Autodesk Inventor part; units mm, degrees
ref_plane "IP_2_XY" through (15.5, 0, 0) normal (1, 0, 0) x (0, 0, -1)
ref_plane "IP_2_YZ" through (15.5, 0, 0) normal (0, 0, -1) x (0, 1, 0)
ref_plane "IP_2_ZX" through (15.5, 0, 0) normal (0, 1, 0) x (1, 0, 0)
sketch "Sketch_1" plane through (0, 0, 0) normal (0, 0, 1) x (1, 0, 0)
  line L0 (50, 0) -> (-50, 0)
  line L1 (0, 23.1136) -> (0, 17.5)
  line L2 (0, 17.5) -> (31, 17.5)
  line L3 (31, 17.5) -> (31, 23.1136)
  line L4 (31, 23.1136) -> (27.7302, 23.1136)
  arc A0 (27.7302, 23.1136) -> (26.8226, 22.8599) centre (27.7302, 21.3636) ccw
  arc A1 (19.6774, 22.8599) -> (26.8226, 22.8599) centre (23.25, 28.75) ccw
  arc A2 (19.6774, 22.8599) -> (18.7698, 23.1136) centre (18.7698, 21.3636) ccw
  line L5 (18.7698, 23.1136) -> (12.2302, 23.1136)
  arc A3 (12.2302, 23.1136) -> (11.3226, 22.8599) centre (12.2302, 21.3636) ccw
  arc A4 (4.1774, 22.8599) -> (11.3226, 22.8599) centre (7.75, 28.75) ccw
  arc A5 (4.1774, 22.8599) -> (3.2698, 23.1136) centre (3.2698, 21.3636) ccw
  line L6 (3.2698, 23.1136) -> (0, 23.1136)
revolve "Revolution1" add sketch "Sketch_1" angle 360 about axis through (50, 0, 0) along (1, 0, 0)
ref_plane "IP_2_XY" through (15.5, 0, 0) normal (1, 0, 0) x (0, 0, -1)
ref_plane "IP_2_YZ" through (15.5, 0, 0) normal (0, 0, -1) x (0, 1, 0)
ref_plane "IP_2_ZX" through (15.5, 0, 0) normal (0, 1, 0) x (1, 0, 0)
ref_plane "IP_3_1_XY" through (7.75, 28.75, 0) normal (1, 0, 0) x (0, 0, -1)
ref_plane "IP_3_1_YZ" through (7.75, 28.75, 0) normal (0, 0, -1) x (0, 1, 0)
ref_plane "IP_3_1_ZX" through (7.75, 28.75, 0) normal (0, 1, 0) x (1, 0, 0)
ref_plane "IP_3_10_XY" through (7.75, 23.2592, -16.8988) normal (1, 0, 0) x (0, 0, -1)
ref_plane "IP_3_10_YZ" through (7.75, 23.2592, -16.8988) normal (0, 0, -1) x (0, 1, 0)
ref_plane "IP_3_10_ZX" through (7.75, 23.2592, -16.8988) normal (0, 1, 0) x (1, 0, 0)
ref_plane "IP_3_2_XY" through (7.75, 23.2592, 16.8988) normal (1, 0, 0) x (0, 0, -1)
ref_plane "IP_3_2_YZ" through (7.75, 23.2592, 16.8988) normal (0, 0, -1) x (0, 1, 0)
ref_plane "IP_3_2_ZX" through (7.75, 23.2592, 16.8988) normal (0, 1, 0) x (1, 0, 0)
ref_plane "IP_3_3_XY" through (7.75, 8.8842, 27.3429) normal (1, 0, 0) x (0, 0, -1)
ref_plane "IP_3_3_YZ" through (7.75, 8.8842, 27.3429) normal (0, 0, -1) x (0, 1, 0)
ref_plane "IP_3_3_ZX" through (7.75, 8.8842, 27.3429) normal (0, 1, 0) x (1, 0, 0)
ref_plane "IP_3_4_XY" through (7.75, -8.8842, 27.3429) normal (1, 0, 0) x (0, 0, -1)
ref_plane "IP_3_4_YZ" through (7.75, -8.8842, 27.3429) normal (0, 0, -1) x (0, 1, 0)
ref_plane "IP_3_4_ZX" through (7.75, -8.8842, 27.3429) normal (0, 1, 0) x (1, 0, 0)
ref_plane "IP_3_5_XY" through (7.75, -23.2592, 16.8988) normal (1, 0, 0) x (0, 0, -1)
ref_plane "IP_3_5_YZ" through (7.75, -23.2592, 16.8988) normal (0, 0, -1) x (0, 1, 0)
ref_plane "IP_3_5_ZX" through (7.75, -23.2592, 16.8988) normal (0, 1, 0) x (1, 0, 0)
ref_plane "IP_3_6_XY" through (7.75, -28.75, 0) normal (1, 0, 0) x (0, 0, -1)
ref_plane "IP_3_6_YZ" through (7.75, -28.75, 0) normal (0, 0, -1) x (0, 1, 0)
ref_plane "IP_3_6_ZX" through (7.75, -28.75, 0) normal (0, 1, 0) x (1, 0, 0)
ref_plane "IP_3_7_XY" through (7.75, -23.2592, -16.8988) normal (1, 0, 0) x (0, 0, -1)
ref_plane "IP_3_7_YZ" through (7.75, -23.2592, -16.8988) normal (0, 0, -1) x (0, 1, 0)
ref_plane "IP_3_7_ZX" through (7.75, -23.2592, -16.8988) normal (0, 1, 0) x (1, 0, 0)
ref_plane "IP_3_8_XY" through (7.75, -8.8842, -27.3429) normal (1, 0, 0) x (0, 0, -1)
ref_plane "IP_3_8_YZ" through (7.75, -8.8842, -27.3429) normal (0, 0, -1) x (0, 1, 0)
ref_plane "IP_3_8_ZX" through (7.75, -8.8842, -27.3429) normal (0, 1, 0) x (1, 0, 0)
ref_plane "IP_3_9_XY" through (7.75, 8.8842, -27.3429) normal (1, 0, 0) x (0, 0, -1)
ref_plane "IP_3_9_YZ" through (7.75, 8.8842, -27.3429) normal (0, 0, -1) x (0, 1, 0)
ref_plane "IP_3_9_ZX" through (7.75, 8.8842, -27.3429) normal (0, 1, 0) x (1, 0, 0)
ref_plane "IP_4_1_XY" through (23.25, 27.3429, 8.8842) normal (1, 0, 0) x (0, 0, -1)
ref_plane "IP_4_1_YZ" through (23.25, 27.3429, 8.8842) normal (0, 0, -1) x (0, 1, 0)
ref_plane "IP_4_1_ZX" through (23.25, 27.3429, 8.8842) normal (0, 1, 0) x (1, 0, 0)
ref_plane "IP_4_10_XY" through (23.25, 27.3429, -8.8842) normal (1, 0, 0) x (0, 0, -1)
ref_plane "IP_4_10_YZ" through (23.25, 27.3429, -8.8842) normal (0, 0, -1) x (0, 1, 0)
ref_plane "IP_4_10_ZX" through (23.25, 27.3429, -8.8842) normal (0, 1, 0) x (1, 0, 0)
ref_plane "IP_4_2_XY" through (23.25, 16.8988, 23.2592) normal (1, 0, 0) x (0, 0, -1)
ref_plane "IP_4_2_YZ" through (23.25, 16.8988, 23.2592) normal (0, 0, -1) x (0, 1, 0)
ref_plane "IP_4_2_ZX" through (23.25, 16.8988, 23.2592) normal (0, 1, 0) x (1, 0, 0)
ref_plane "IP_4_3_XY" through (23.25, 0, 28.75) normal (1, 0, 0) x (0, 0, -1)
ref_plane "IP_4_3_YZ" through (23.25, 0, 28.75) normal (0, 0, -1) x (0, 1, 0)
ref_plane "IP_4_3_ZX" through (23.25, 0, 28.75) normal (0, 1, 0) x (1, 0, 0)
ref_plane "IP_4_4_XY" through (23.25, -16.8988, 23.2592) normal (1, 0, 0) x (0, 0, -1)
ref_plane "IP_4_4_YZ" through (23.25, -16.8988, 23.2592) normal (0, 0, -1) x (0, 1, 0)
ref_plane "IP_4_4_ZX" through (23.25, -16.8988, 23.2592) normal (0, 1, 0) x (1, 0, 0)
ref_plane "IP_4_5_XY" through (23.25, -27.3429, 8.8842) normal (1, 0, 0) x (0, 0, -1)
ref_plane "IP_4_5_YZ" through (23.25, -27.3429, 8.8842) normal (0, 0, -1) x (0, 1, 0)
ref_plane "IP_4_5_ZX" through (23.25, -27.3429, 8.8842) normal (0, 1, 0) x (1, 0, 0)
ref_plane "IP_4_6_XY" through (23.25, -27.3429, -8.8842) normal (1, 0, 0) x (0, 0, -1)
ref_plane "IP_4_6_YZ" through (23.25, -27.3429, -8.8842) normal (0, 0, -1) x (0, 1, 0)
ref_plane "IP_4_6_ZX" through (23.25, -27.3429, -8.8842) normal (0, 1, 0) x (1, 0, 0)
ref_plane "IP_4_7_XY" through (23.25, -16.8988, -23.2592) normal (1, 0, 0) x (0, 0, -1)
ref_plane "IP_4_7_YZ" through (23.25, -16.8988, -23.2592) normal (0, 0, -1) x (0, 1, 0)
ref_plane "IP_4_7_ZX" through (23.25, -16.8988, -23.2592) normal (0, 1, 0) x (1, 0, 0)
ref_plane "IP_4_8_XY" through (23.25, 0, -28.75) normal (1, 0, 0) x (0, 0, -1)
ref_plane "IP_4_8_YZ" through (23.25, 0, -28.75) normal (0, 0, -1) x (0, 1, 0)
ref_plane "IP_4_8_ZX" through (23.25, 0, -28.75) normal (0, 1, 0) x (1, 0, 0)
ref_plane "IP_4_9_XY" through (23.25, 16.8988, -23.2592) normal (1, 0, 0) x (0, 0, -1)
ref_plane "IP_4_9_YZ" through (23.25, 16.8988, -23.2592) normal (0, 0, -1) x (0, 1, 0)
ref_plane "IP_4_9_ZX" through (23.25, 16.8988, -23.2592) normal (0, 1, 0) x (1, 0, 0)
properties part number "hpc_Q2307-ACC_2"
Work out the finished part from the listing and answer in its coordinate system (mm). Give positions to 0.01 mm unless a question says otherwise; leave off trailing zeros. Write each loop counter-clockwise with the first axis right and the second up, starting at its lowest first coordinate (ties: lowest second). Pieces come first, ordered by that corner, then holes.
(1) The part is cut by section C-C on x = 16. Write down the section's boundary in (y, z).
Final values:
outline: circle Ø46.23 at (0, 0); hole circle Ø35 at (0, 0)
(2) The mould has two halves that part along Y. Classify faces 1 (the flat face through (31, 8, 16)), 2 (the cylindrical face through (29.342, -5.011, 22.564)), 3 (the cylindrical face through (15.717, -13.887, -10.648)): pulls with the +Y half, pulls with the -Y half, needs draft (parallel to the pull), parting line crosses it, or undercut.
Final values:
face 1: needs draft
face 2: parting line crosses it
face 3: undercut
(3) The part is cut by section A-A on y = 0. Write down the section's boundary in (x, z).
Final values:
outline: (0, -23.11) - (3.27, -23.11) arc R1.75 ccw to (4.18, -22.86) arc R6.89 cw to (11.32, -22.86) arc R1.75 ccw to (12.23, -23.11) - (18.77, -23.11) arc R1.75 ccw to (19.68, -22.86) arc R6.89 cw to (26.82, -22.86) arc R1.75 ccw to (27.73, -23.11) - (31, -23.11) - (31, -17.5) - (0, -17.5) - close; (0, 17.5) - (31, 17.5) - (31, 23.11) - (27.73, 23.11) arc R1.75 ccw to (26.82, 22.86) arc R6.89 cw to (19.68, 22.86) arc R1.75 ccw to (18.77, 23.11) - (12.23, 23.11) arc R1.75 ccw to (11.32, 22.86) arc R6.89 cw to (4.18, 22.86) arc R1.75 ccw to (3.27, 23.11) - (0, 23.11) - close
(4) The part is cut by section D-D on x = 6.5. Write down the section's boundary in (y, z), plus the area to 3 significant figures.
Final values:
outline: circle Ø43.95 at (0, 0); hole circle Ø35 at (0, 0)
area: 555 mm2
(5) Flat-ended cylindrical pins translate along their axes: pin 1 Ø5 at (x, y) = (21.5, 15.5) entering from +Z; pin 2 Ø4 at (x, y) = (9.5, -9) entering from -Z; pin 3 Ø6 at (x, z) = (18.5, 9.5) entering from +Y; pin 4 Ø10 at (x, z) = (14, 3.5) entering from +Y. Find the tip coordinate at first contact, or state that the pin passes through.
Final values:
pin 1: stops at z = 18.23
pin 2: stops at z = -21.36
pin 3: stops at y = 22.18
pin 4: stops at y = 23.11
(6) Straight lines are drawn through the part: line 1 (Z direction, x = 13.5, y = 0); line 2 (X direction, y = -16.5, z = -16); line 3 (Y direction, x = 17, z = -3.5). For each, find the intervals that lie inside material, in ascending order.
Final values:
line 1: z = -23.11 to -17.5, 17.5 to 23.11
line 2: x = 0 to 3.93, 11.57 to 19.43, 27.07 to 31
line 3: y = -22.85 to -17.15, 17.15 to 22.85
